Read the model definition and answer for the solid it produces. Units are mm, in the model's axes. Round coordinates to 2 decimals unless told otherwise and drop trailing zeros. Order: outer loops, then holes, each group sorted by start corner. A loop starts at its lowest first (then second) coordinate and runs counter-clockwise, first axis right, second up.
from build123d import *

# Parameters (mm, degrees)
SKETCH1_R           = 1.5
SKETCH1_R_2         = 2.5
BOSS_EXTRUDE2_DEPTH = 6
FILLET1_R           = 3


with BuildPart() as part:
    # Sketch1 → Boss-Extrude2 (new body)
    with BuildSketch(Plane.XY):
        Polygon((20.766769668, -12.307033049), (0.274818432, 24.138066612), (-21.0415881, -11.831033562), align=None)
        with Locations((0.173413232, 16.164877395)):
            Circle(SKETCH1_R, mode=Mode.SUBTRACT)
        with Locations((13.912487857, -8.232618961)):
            Circle(SKETCH1_R, mode=Mode.SUBTRACT)
        with Locations((-14.085901089, -7.932258433)):
            Circle(SKETCH1_R, mode=Mode.SUBTRACT)
        Circle(SKETCH1_R_2, mode=Mode.SUBTRACT)
    extrude(amount=BOSS_EXTRUDE2_DEPTH)

    # Fillet1
    fillet1_edges = [part.edges().sort_by_distance(p)[0] for p in [
        (0.274818432, 24.138066612, 3),
        (20.766769668, -12.307033049, 3),
        (-21.0415881, -11.831033562, 3),
    ]]
    fillet(fillet1_edges, radius=FILLET1_R)


solid = part.part
Q1. A cutting plane is placed at A-A, the plane x = 0. Give the vertices of the cut face in (y, z).
Outcome:
outline: (-12.07, 0) - (-2.5, 0) - (-2.5, 6) - (-12.07, 6) - close; (2.5, 0) - (14.67, 0) - (14.67, 6) - (2.5, 6) - close; (17.65, 0) - (21.13, 0) - (21.13, 6) - (17.65, 6) - close
Q2. Flat-ended cylindrical pins translate along their axes: pin 1 (1 mm diameter, centred on y = 4, z = 3.5, fed in from +X); pin 2 (1 mm diameter, centred on x = 14, z = 3.5, fed in from +Y); pin 3 (1.5 mm diameter, centred on x = 5, z = 1.5, fed in from -Y). Find the tip coordinate at first contact, or state that the pin passes through.
Outcome:
pin 1: stops at x = 11.88
pin 2: stops at y = 0.62
pin 3: stops at y = -12.14
Q3. Straight lines are drawn through the part: probe 1 along X at (y, z) = (-8, 5); probe 2 along Y at (x, z) = (0, 1.65); probe 3 along X at (y, z) = (17, 4). For each, find the intervals that lie inside material, in ascending order.
Outcome:
probe 1: x = -18.68 to -15.58, -12.59 to 12.43, 15.39 to 18.33
probe 2: y = -12.07 to -2.5, 2.5 to 14.67, 17.65 to 21.13
probe 3: x = -3.96 to -1.07, 1.42 to 4.29
Q4. A cutting plane is placed at C-C, the plane y = 0. Give the vertices of the cut face in (x, z), plus the area to 3 significant figures.
Outcome:
outline: (-14.03, 0) - (-2.5, 0) - (-2.5, 6) - (-14.03, 6) - close; (2.5, 0) - (13.85, 0) - (13.85, 6) - (2.5, 6) - close
area: 137 mm2
Q5. For a pull along X with two mould halves and no side action, classify faces 1 (the face through (10.63, 5.72, 2.96)), 2 (the face through (12.722, -9.145, 2.958)), 3 (the face through (-18.405, -10.399, 3.042)) as released by +X, released by -X, zero draft, split by the parting line, or undercut.
Outcome:
face 1: released by +X
face 2: undercut
face 3: released by -X
Q6. A cutting plane is placed at B-B, the plane z = 5.3. Give the vertices of the cut face in (x, y).
Outcome:
outline: (-18.39, -7.36) arc R3 ccw to (-15.85, -11.89) - (15.57, -12.25) arc R3 ccw to (18.22, -7.78) - (2.82, 19.61) arc R3 ccw to (-2.37, 19.67) - close; hole circle Ø3 at (-14.09, -7.93); hole circle Ø5 at (0, 0); hole circle Ø3 at (0.17, 16.16); hole circle Ø3 at (13.91, -8.23)
Q7. A cutting plane is placed at D-D, the plane x = 4. Give the vertices of the cut face in (y, z), plus the area to 3 significant figures.
Outcome:
outline: (-12.12, 0) - (17.51, 0) - (17.51, 6) - (-12.12, 6) - close
area: 178 mm2
